Input: part model. Units: mm. Frame: model coordinates. Round coordinates to 2 decimals unless told otherwise and drop trailing zeros. Order: outer loops, then holes, each group sorted by start corner. A loop starts at its lowest first (then second) coordinate and runs counter-clockwise, first axis right, second up.
Item 1: Cut plane C-C on y = 4. Output: boundary loops of the cut face in (x, z), then the cut area to 3 significant figures.
Item 2: Cut plane A-A on x = 51. Output: boundary loops of the cut face in (y, z).
Item 3: Cut plane D-D on z = 42.85. Output: boundary loops of the cut face in (x, y).
Item 4: Line query: L1, parallel to X at y = 39, z = 42.55; L2, parallel to Y at x = 48, z = 41.95; L3, parallel to Y at x = 51, z = 42.2. Output: solid intervals per line, ascending.
Item 5: Cut plane B-B on y = 12. Output: boundary loops of the cut face in (x, z), then the cut area to 3 significant figures.
```python
from build123d import *

# Parameters (mm, degrees)
CYLINDER004_R     = 2
CYLINDER004_DEPTH = 10
CYLINDER005_R     = 2
CYLINDER005_DEPTH = 10
CYLINDER006_R     = 2
CYLINDER006_DEPTH = 10
CYLINDER003_R     = 2
CYLINDER003_DEPTH = 10
SKETCH001_W       = 60
SKETCH001_H       = 43
SKETCH001_R       = 1.5
SKETCH001_W_2     = 48
SKETCH001_H_2     = 10
EXTRUDE001_DEPTH  = 3


with BuildPart() as cylinder004:
    # Cylinder004 → Cylinder004 (new body)
    with BuildSketch(Plane(origin=(5, 39, 40), x_dir=(1, 0, 0), z_dir=(0, 0, 1))):
        Circle(CYLINDER004_R)
    extrude(amount=CYLINDER004_DEPTH)


with BuildPart() as cylinder005:
    # Cylinder005 → Cylinder005 (new body)
    with BuildSketch(Plane(origin=(51, 39, 40), x_dir=(1, 0, 0), z_dir=(0, 0, 1))):
        Circle(CYLINDER005_R)
    extrude(amount=CYLINDER005_DEPTH)


with BuildPart() as cylinder006:
    # Cylinder006 → Cylinder006 (new body)
    with BuildSketch(Plane(origin=(51, 4, 40), x_dir=(1, 0, 0), z_dir=(0, 0, 1))):
        Circle(CYLINDER006_R)
    extrude(amount=CYLINDER006_DEPTH)


with BuildPart() as fusion008:
    # Cylinder003 → Cylinder003 (new body)
    with BuildSketch(Plane(origin=(5, 4, 40), x_dir=(1, 0, 0), z_dir=(0, 0, 1))):
        Circle(CYLINDER003_R)
    extrude(amount=CYLINDER003_DEPTH)

    # Fusion008: union Cylinder004, Cylinder005, Cylinder006
    add(cylinder004.part)
    add(cylinder005.part)
    add(cylinder006.part)


with BuildPart() as cut004:
    # Sketch001 → Extrude001 (new body)
    with BuildSketch(Plane.XY):
        with Locations((-30, 21.5)):
            Rectangle(SKETCH001_W, SKETCH001_H)
        with Locations((-55, 21.5)):
            Circle(SKETCH001_R, mode=Mode.SUBTRACT)
        with Locations((-30, 12.5)):
            Rectangle(SKETCH001_W_2, SKETCH001_H_2, mode=Mode.SUBTRACT)
        with Locations((-30, 30.5)):
            Rectangle(SKETCH001_W_2, SKETCH001_H_2, mode=Mode.SUBTRACT)
    extrude(amount=EXTRUDE001_DEPTH)


with BuildPart() as cut004_1:
    # Extrude001 placement: moved
    add(cut004.part.moved(Location((58, 0, 41.5))))

    # Cut004: cut Fusion008
    add(fusion008.part, mode=Mode.SUBTRACT)


solid = cut004_1.part
```
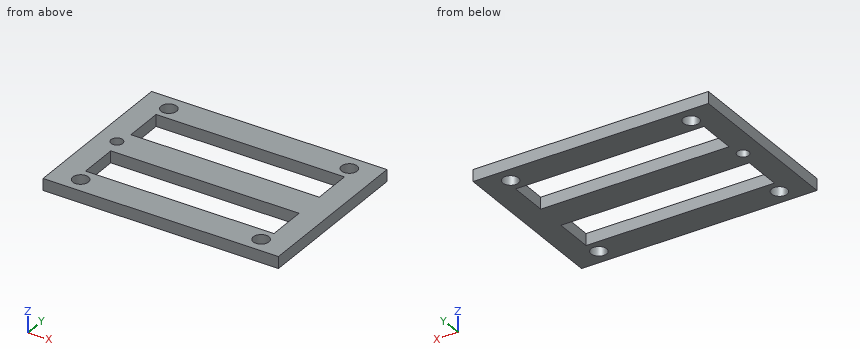
From the geometry:
1. outline: (-2, 41.5) - (3, 41.5) - (3, 44.5) - (-2, 44.5) - close; (7, 41.5) - (49, 41.5) - (49, 44.5) - (7, 44.5) - close; (53, 41.5) - (58, 41.5) - (58, 44.5) - (53, 44.5) - close
1. area: 156 mm2
2. outline: (0, 41.5) - (2, 41.5) - (2, 44.5) - (0, 44.5) - close; (6, 41.5) - (7.5, 41.5) - (7.5, 44.5) - (6, 44.5) - close; (17.5, 41.5) - (25.5, 41.5) - (25.5, 44.5) - (17.5, 44.5) - close; (35.5, 41.5) - (37, 41.5) - (37, 44.5) - (35.5, 44.5) - close; (41, 41.5) - (43, 41.5) - (43, 44.5) - (41, 44.5) - close
3. outline: (-2, 0) - (58, 0) - (58, 43) - (-2, 43) - close; hole circle Ø3 at (3, 21.5); hole circle Ø4 at (5, 4); hole circle Ø4 at (5, 39); hole (4, 7.5) - (52, 7.5) - (52, 17.5) - (4, 17.5) - close; hole (4, 25.5) - (52, 25.5) - (52, 35.5) - (4, 35.5) - close; hole circle Ø4 at (51, 4); hole circle Ø4 at (51, 39)
4. L1: x = -2 to 3, 7 to 49, 53 to 58
4. L2: y = 0 to 7.5, 17.5 to 25.5, 35.5 to 43
4. L3: y = 0 to 2, 6 to 7.5, 17.5 to 25.5, 35.5 to 37, 41 to 43
5. outline: (-2, 41.5) - (4, 41.5) - (4, 44.5) - (-2, 44.5) - close; (52, 41.5) - (58, 41.5) - (58, 44.5) - (52, 44.5) - close
5. area: 36.0 mm2
